Drawing for the job (mm, zero at the part's lowest x, y, z). Give positions to 0.01 mm unless a question says otherwise; leave off trailing zeros. Loops run counter-clockwise (first coordinate to the right, second up) from the corner with the lowest first, then second, coordinate; pieces in that order, holes last.
1) Band-saw the part on A-A on x = 23.5. List the corners of the cut face in (y, z), then the cut area to 3 significant figures.
2) Two-plate mould, pull along X, no slides. Class the marked faces 1, 2, 3 and 4: +X half, -X half, draft (parallel to the pull), parting line (faces both ways), or undercut.
3) Band-saw the part on D-D on z = 2.25. List the corners of the cut face in (x, y).
4) Band-saw the part on C-C on z = 7.5. List the corners of the cut face in (x, y).
5) Wall check: line 1 (X direction, y = 2.75, z = 13); line 2 (X direction, y = 2.75, z = 5.5); line 3 (X direction, y = 1.05, z = 1.25). Give the ranges that are in metal, low to high.
6) Band-saw the part on B-B on y = 2.75. List the corners of the cut face in (x, z).
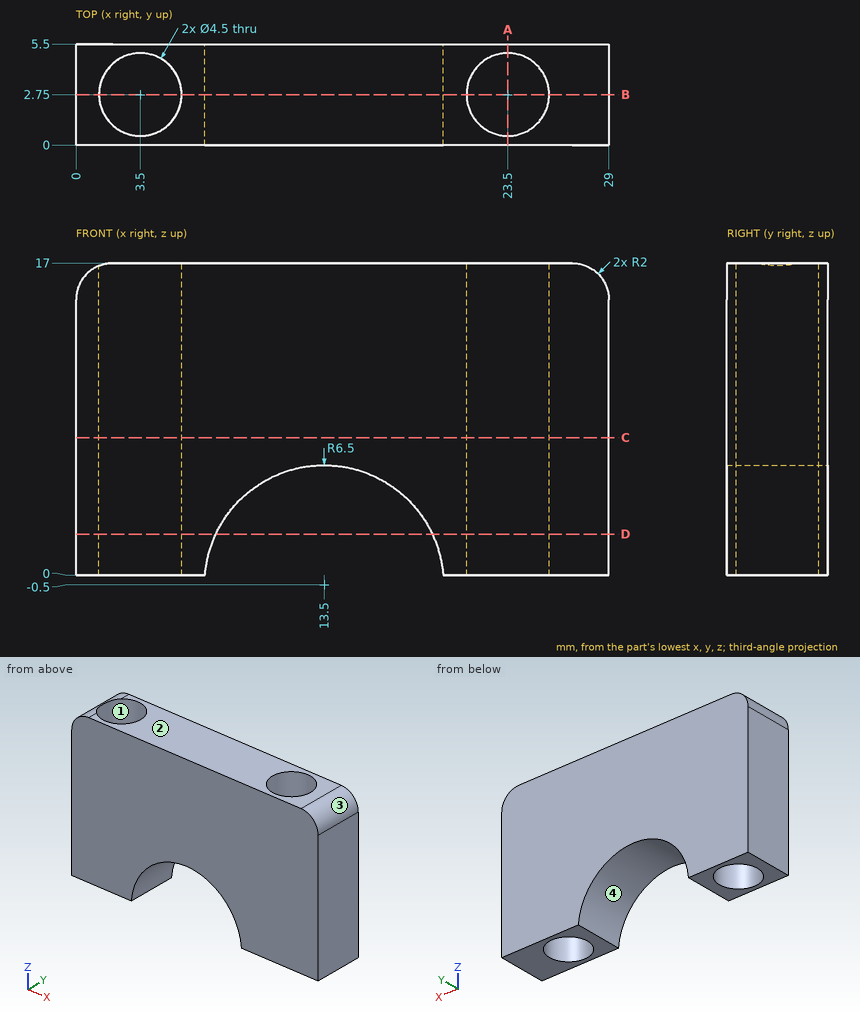
Findings below:
1. outline: (0, 0) - (0.5, 0) - (0.5, 17) - (0, 17) - close; (5, 0) - (5.5, 0) - (5.5, 17) - (5, 17) - close
1. area: 17.0 mm2
2. face 1: undercut
2. face 2: draft
2. face 3: +X half
2. face 4: undercut
3. outline: (0, 0) - (7.61, 0) - (7.61, 5.5) - (0, 5.5) - close; (19.39, 0) - (29, 0) - (29, 5.5) - (19.39, 5.5) - close; hole circle Ø4.5 at (3.5, 2.75); hole circle Ø4.5 at (23.5, 2.75)
4. outline: (0, 0) - (29, 0) - (29, 5.5) - (0, 5.5) - close; hole circle Ø4.5 at (3.5, 2.75); hole circle Ø4.5 at (23.5, 2.75)
5. line 1: x = 0 to 1.25, 5.75 to 21.25, 25.75 to 29
5. line 2: x = 0 to 1.25, 5.75 to 11, 16 to 21.25, 25.75 to 29
5. line 3: x = 0 to 2.03, 4.97 to 7.24, 19.76 to 22.03, 24.97 to 29
6. outline: (0, 0) - (1.25, 0) - (1.25, 16.85) arc R2 ccw to (0, 15) - close; (5.75, 0) - (7.02, 0) arc R6.5 cw to (19.98, 0) - (21.25, 0) - (21.25, 17) - (5.75, 17) - close; (25.75, 0) - (29, 0) - (29, 15) arc R2 ccw to (27, 17) - (25.75, 17) - close
